from build123d import *
from build123d import SkipClean  # not in build123d's __all__

# Parameters (mm, degrees)
F1_DEPTH = 65
F2_R     = 40.5
F2_R_2   = 21.5
F3_DEPTH = 11.5
F4_R     = 40.5
F4_R_2   = 21.5
F5_DEPTH = 11.5
F7_D     = 14
F9_R     = 10
F10_D    = 16


# Not quite as in the source:
# - after a boolean that leaves OpenCascade's solid faulty, fix() repairs it


with BuildPart() as f1:
    # F0 (on Front) → F1 (new body)
    with BuildSketch(Plane.XZ):
        with BuildLine():
            Line((0, 16), (0, 0))
            Line((0, 0), (101.5, 0))
            Line((101.5, 0), (101.5, 16))
            Line((101.5, 16), (67, 16))
            ThreePointArc((67, 16), (52.2079138911, 37.4608144218), (47, 63))
            ThreePointArc((47, 63), (33.2340187158, 96.2340187158), (0, 110))
            Line((0, 110), (0, 84.5))
            ThreePointArc((0, 84.5), (15.2027957955, 78.2027957955), (21.5, 63))
            ThreePointArc((21.5, 63), (15.2027957955, 47.7972042045), (0, 41.5))
            Line((0, 41.5), (0, 16))
        make_face()
        with BuildLine():
            Line((-101.5, 0), (0, 0))
            Line((0, 0), (0, 16))
            Line((0, 16), (0, 41.5))
            ThreePointArc((0, 41.5), (-21.5, 63), (0, 84.5))
            Line((0, 84.5), (0, 110))
            ThreePointArc((0, 110), (-33.2340187158, 96.2340187158), (-47, 63))
            ThreePointArc((-47, 63), (-52.2079138911, 37.4608144218), (-67, 16))
            Line((-67, 16), (-101.5, 16))
            Line((-101.5, 16), (-101.5, 0))
        make_face()
    extrude(amount=F1_DEPTH)

    # F2 (on face) → F3 (join)
    with BuildSketch(Plane.XZ.offset(65)):
        with Locations((0, 63)):
            Circle(F2_R)
        with Locations((0, 63)):
            Circle(F2_R_2, mode=Mode.SUBTRACT)
    extrude(amount=F3_DEPTH)

    # F4 (on face) → F5 (join)
    with BuildSketch(Plane(origin=(0, 0, 0), x_dir=(-1, 0, 0), z_dir=(0, 1, 0))):
        with Locations((0, 63)):
            Circle(F4_R)
        with Locations((0, 63)):
            Circle(F4_R_2, mode=Mode.SUBTRACT)
    with SkipClean():  # cleaning this boolean's faces spoils the solid; the shape is the same uncleaned
        extrude(amount=F5_DEPTH)

    # F7 (through all)
    with Locations(Plane.XY.offset(16)):
        with Locations((84.25, -32.5)):
            Hole(F7_D / 2)

    add(f1.part.fix(), mode=Mode.REPLACE)

    # F9
    f9_edges = [f1.edges().sort_by_distance(p)[0] for p in [
        (-67, -32.5, 16),
        (67, -32.5, 16),
    ]]
    fillet(f9_edges, radius=F9_R)

    # F10 (through all)
    with Locations(Plane.XY.offset(16)):
        with Locations((-84.25, -32.5)):
            Hole(F10_D / 2)


solid = f1.part
Input: part model. Units: mm. Frame: model coordinates. A direction names the side the tool comes from. Coordinates: 2 decimals unless noted, no trailing zeros. Order: outer loops, then holes, each group sorted by start corner. A loop starts at its lowest first (then second) coordinate and runs counter-clockwise, first axis right, second up. Notation, with made-up numbers: M 6.5,44.25 L 50.5,44.25 A11 cw 50.5,54.25 Z; hole C 11.25,55 d10. An arc over 180 degrees is marked long. Answer in a Markdown table with one row per item.
(1) Section query A-A, the plane y = -32.5. Output: boundary loops of the cut face in (x, z) (3 decimals).
Numbers:
| item | result |
|---|---|
| outline | M -101.5,0 L -92.25,0 L -92.25,16 L -101.5,16 Z; M -76.25,0 L 77.25,0 L 77.25,16 L 71.227,16 A10 cw 63.804,19.3 A65.225 cw 47,63 A47 ccw -47,63 A65.225 cw -63.804,19.3 A10 cw -71.227,16 L -76.25,16 Z; M 91.25,0 L 101.5,0 L 101.5,16 L 91.25,16 Z; hole C 0,63 d43 |
(2) Draft query along Y for faces 4 (the cylindrical face through (-8.78, -70.67, 23.463)), 5 (the flat face through (17, -76.5, 46)), 6 (the flat face through (0, 0, 19)), 7 (the cylindrical face through (91.243, -32.192, 7.888)). Return one class per face: pulls with the +Y half, pulls with the -Y half, needs draft (parallel to the pull), parting line crosses it, or undercut.
Numbers:
| item | result |
|---|---|
| face 4 | needs draft |
| face 5 | pulls with the -Y half |
| face 6 | pulls with the +Y half |
| face 7 | undercut |
(3) Access query for faces 1 (the cylindrical face through (8.78, 5.67, 23.463)), 2 (the flat face through (-93, -32, 16)), 3 (the flat face through (93, -32, 16)). Directions: +Z, -Z, +X, -X, +Y, -Y. A direction counts if a zero-diameter tool reaches every point of the face in a straight line with its end or side. Return the directions, or none.
Numbers:
| item | result |
|---|---|
| face 1 | +Y |
| face 2 | +Z, -X, +Y, -Y |
| face 3 | +Z, +X, +Y, -Y |
(4) Section query D-D, the plane z = 53.5. Output: boundary loops of the cut face in (x, y), plus the area to 3 significant figures.
Numbers:
| item | result |
|---|---|
| outline | M -47.7,-65 L -39.37,-65 L -39.37,-76.5 L -19.29,-76.5 L -19.29,11.5 L -39.37,11.5 L -39.37,0 L -47.7,0 Z; M 19.29,-76.5 L 39.37,-76.5 L 39.37,-65 L 47.7,-65 L 47.7,0 L 39.37,0 L 39.37,11.5 L 19.29,11.5 Z |
| area | 4,620 mm^2 |
(5) Material intervals for line 1 (X direction, y = -32, z = 13); line 2 (X direction, y = -40, z = 64); line 3 (Z direction, x = 0, y = 7.75), sorted ascending. Write a range as [from, to].
Numbers:
| item | result |
|---|---|
| line 1 | x = [-101.5, -92.23], [-76.27, 77.27], [91.23, 101.5] |
| line 2 | x = [-46.99, -21.48], [21.48, 46.99] |
| line 3 | z = [22.5, 41.5], [84.5, 103.5] |
(6) Section query C-C, the plane y = -50. Output: boundary loops of the cut face in (x, z) (3 decimals), plus the area to 3 significant figures.
Numbers:
| item | result |
|---|---|
| outline | M -101.5,0 L 101.5,0 L 101.5,16 L 71.227,16 A10 cw 63.804,19.3 A65.225 cw 47,63 A47 ccw -47,63 A65.225 cw -63.804,19.3 A10 cw -71.227,16 L -101.5,16 Z; hole C 0,63 d43 |
| area | 10,300 mm^2 |
(7) Section query B-B, the plane x = 84.25. Output: boundary loops of the cut face in (y, z), plus the area to 3 significant figures.
Numbers:
| item | result |
|---|---|
| outline | M -65,0 L -39.5,0 L -39.5,16 L -65,16 Z; M -25.5,0 L 0,0 L 0,16 L -25.5,16 Z |
| area | 816 mm^2 |
(8) Contact query for flat-ended pins moving along their axis: pin 1 Ø1.5 at (x, y) = (66.5, -37.5) entering from +Z; pin 2 Ø2 at (x, z) = (-27.5, 21.5) entering from -Y; pin 3 Ø11 at (x, y) = (84.25, -32.5) entering from +Z; pin 4 Ø24 at (x, y) = (-85, -31) entering from +Z. Output: stop coordinate, or through.
Numbers:
| item | result |
|---|---|
| pin 1 | stops at z = 17.63 |
| pin 2 | stops at y = -65 |
| pin 3 | passes through |
| pin 4 | stops at z = 16 |
